Verification items for this drawing (mm, ordinates from the low corner). Round coordinates to 2 decimals unless told otherwise and drop trailing zeros. Loops run counter-clockwise (first coordinate to the right, second up) from the corner with the lowest first, then second, coordinate; pieces in that order, holes last. Notation, with made-up numbers: (86, -15.75) -> (101, -15.75) arc R20 cw to (101, 6.25) -> close; hole circle Ø11 at (27.25, 56). An arc over 180 degrees is marked (long way). One line per question, with ' | ' between items.
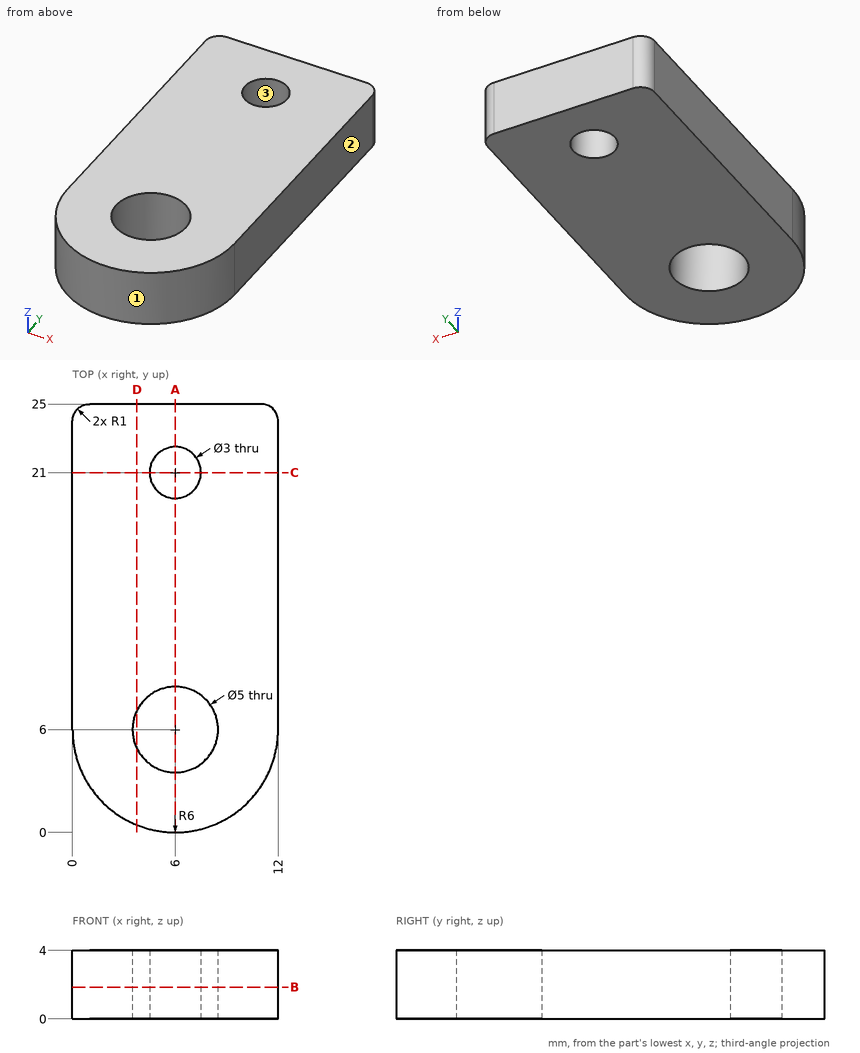
(1) Scan lines: probe 1 along Y at (x, z) = (6, 1.55); probe 2 along X at (y, z) = (6.5, 0.85); probe 3 along Y at (x, z) = (8, 2). Record each from-to range of solid material in increasing order.
Answer:
probe 1: y = 0 to 3.5, 8.5 to 19.5, 22.5 to 25 | probe 2: x = 0 to 3.55, 8.45 to 12 | probe 3: y = 0.34 to 4.5, 7.5 to 25
(2) Go/stop test with flat-tipped pins: pin 1 (1 mm diameter, centred on x = 5, z = 2, fed in from -Y); pin 2 (4 mm diameter, centred on x = 6, y = 21, fed in from +Z); pin 3 (1.5 mm diameter, centred on x = 3, z = 1.5, fed in from -Y). Record where each tip stops, or that it passes through.
Answer:
pin 1: stops at y = 0.02 | pin 2: stops at z = 4 | pin 3: stops at y = 0.44
(3) Sectioned sample at D-D, the plane x = 3.75. Record the cut outline in (y, z).
Answer:
outline: (0.44, 0) -> (4.91, 0) -> (4.91, 4) -> (0.44, 4) -> close; (7.09, 0) -> (25, 0) -> (25, 4) -> (7.09, 4) -> close
(4) Sectioned sample at B-B, the plane z = 1.85. Record the cut outline in (x, y).
Answer:
outline: (0, 6) arc R6 ccw to (12, 6) -> (12, 24) arc R1 ccw to (11, 25) -> (1, 25) arc R1 ccw to (0, 24) -> close; hole circle Ø5 at (6, 6); hole circle Ø3 at (6, 21)
(5) Sectioned sample at C-C, the plane y = 21. Record the cut outline in (x, z).
Answer:
outline: (0, 0) -> (4.5, 0) -> (4.5, 4) -> (0, 4) -> close; (7.5, 0) -> (12, 0) -> (12, 4) -> (7.5, 4) -> close
(6) Sectioned sample at A-A, the plane x = 6. Record the cut outline in (y, z).
Answer:
outline: (0, 0) -> (3.5, 0) -> (3.5, 4) -> (0, 4) -> close; (8.5, 0) -> (19.5, 0) -> (19.5, 4) -> (8.5, 4) -> close; (22.5, 0) -> (25, 0) -> (25, 4) -> (22.5, 4) -> close
(7) Mould release check, pull along Y, two halves, no side actions. Record for the marked faces 1, 2 and 3: +Y half, -Y half, draft (parallel to the pull), parting line (faces both ways), or undercut.
Answer:
face 1: -Y half | face 2: draft | face 3: undercut
